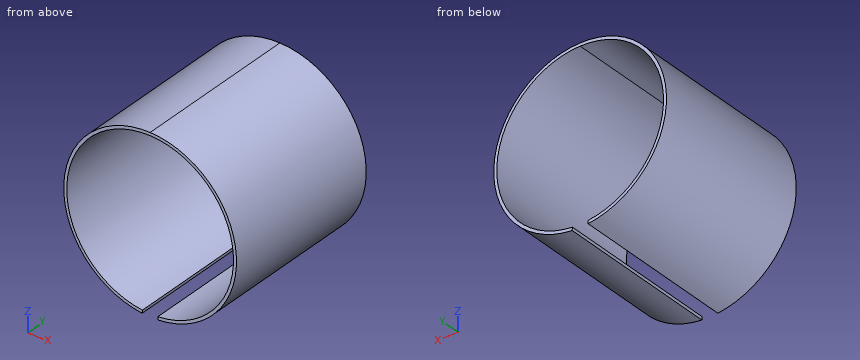
from build123d import *

# Parameters (mm, degrees)
SKETCH_1_R               = 86.5
SKETCH_1_R_2             = 83.5
EXTRUDE_1_DEPTH          = 165.5
CUT_EXTRUDE_1_DEPTH      = 206.802696775
CUT_EXTRUDE_1_DEPTH_BACK = 206.802696775


with BuildPart() as part:
    # Эскиз1 → Бобышка-Вытянуть1 (new body)
    with BuildSketch(Plane(origin=(0, 0, 0), x_dir=(1, 0, 0), z_dir=(0, 1, 0))):
        with Locations(Location((0, 0, 0), (0, 0, 270))):
            Circle(SKETCH_1_R)
        with Locations(Location((0, 0, 0), (0, 0, 270))):
            Circle(SKETCH_1_R_2, mode=Mode.SUBTRACT)
    extrude(amount=EXTRUDE_1_DEPTH)

    # Эскиз2 → Вырез-Вытянуть1 (cut, two sides: drawn at the far end of the back side and taken through both)
    with BuildSketch(Plane(origin=(0, 165.5, 0), x_dir=(1, 0, 0), z_dir=(0, 1, 0)).offset(-CUT_EXTRUDE_1_DEPTH_BACK)):
        with BuildLine():
            Line((-8, 86.12926332), (-7.722543353, 83.142121239))
            ThreePointArc((-7.722543353, 83.142121239), (0, 83.5), (7.722543353, 83.142121239))
            Line((7.722543353, 83.142121239), (8, 86.12926332))
            ThreePointArc((8, 86.12926332), (0, 86.5), (-8, 86.12926332))
        make_face()
    extrude(amount=CUT_EXTRUDE_1_DEPTH + CUT_EXTRUDE_1_DEPTH_BACK, mode=Mode.SUBTRACT)


solid = part.part
For this review, take the finished solid that the model builds, in its own axes (mm). Give positions to 0.01 mm unless a question says otherwise; leave off trailing zeros. Loops run counter-clockwise (first coordinate to the right, second up) from the corner with the lowest first, then second, coordinate; pieces in that order, holes last. Notation, with made-up numbers: (74, -15.75) - (105, -15.75) arc R6 cw to (105, -4.75) - close; hole circle Ø8 at (-32.5, 4). An arc over 180 degrees is marked (long way). Write each question's results on one line, items separated by ' | '.
(1) Take a section at A-A (z = 0). Give the boundary of the cut face in (x, y), then the cut area to 3 significant figures.
Conclusion:
outline: (-86.5, 0) - (-83.5, 0) - (-83.5, 165.5) - (-86.5, 165.5) - close; (83.5, 0) - (86.5, 0) - (86.5, 165.5) - (83.5, 165.5) - close | area: 993 mm^2
(2) For line 1 along X through (y, z) = (69, -1.5); line 2 along Z through (x, y) = (30, 37.5); line 3 along Z through (x, y) = (-28, 24.5), list the stretches that pass through material, from the lowest coordinate up.
Conclusion:
line 1: -86.49 to -83.49, 83.49 to 86.49 | line 2: -81.13 to -77.92, 77.92 to 81.13 | line 3: -81.84 to -78.67, 78.67 to 81.84
(3) For pin 1 Ø6 at (y, z) = (125.5, -26.5) entering from +X; pin 2 Ø1.5 at (x, y) = (64, 111) entering from -Z; pin 3 Ø1.5 at (x, y) = (53, 19) entering from +Z, all flat-tipped, find the tip position at first contact; note any pin that passes through.
Conclusion:
pin 1: x = 83.25 | pin 2: z = -59.01 | pin 3: z = 68.94
(4) Take a section at C-C (y = 12). Give the boundary of the cut face in (x, z), then the cut area to 3 significant figures.
Conclusion:
outline: (-8, -86.13) - (-7.72, -83.14) arc R83.5 cw (long way) to (7.72, -83.14) - (8, -86.13) arc R86.5 ccw (long way) to start | area: 1,550 mm^2
(5) Take a section at B-B (x = 67.5). Give the boundary of the cut face in (y, z), then the cut area to 3 significant figures.
Conclusion:
outline: (0, -54.09) - (165.5, -54.09) - (165.5, -49.15) - (0, -49.15) - close; (0, 49.15) - (165.5, 49.15) - (165.5, 54.09) - (0, 54.09) - close | area: 1,640 mm^2
